Geometry check sheet. Reference: the model listing, model coordinates, mm. Coordinates: 2 decimals unless noted, no trailing zeros. Write each loop counter-clockwise with the first axis right and the second up, starting at its lowest first coordinate (ties: lowest second). Pieces come first, ordered by that corner, then holes. Notation, with made-up numbers: M 56,-0.5 L 77,-0.5 A18 ccw 77,18.5 Z; hole C -11,50 d8. An arc over 180 degrees is marked long. Put each result on its own line as item: value. Start each with the question number.
1) Scan lines: line 1 along Z through (x, y) = (10, -7.25); line 2 along Y through (x, z) = (6.25, 0); line 3 along Y through (x, z) = (7, 0). Record each from-to range of solid material in increasing order.
2) Cross-section at C-C on x = 2.5. Record the cut outline in (y, z), plus the area to 3 significant figures.
3) Gauge pin test, flat ends, axial feed: pin 1 (2 mm diameter, centred on x = 2.5, y = -6, fed in from -Z); pin 2 (3 mm diameter, centred on x = 7, y = -0.5, fed in from -Z); pin 3 (3 mm diameter, centred on x = 5.5, z = 8.5, fed in from -Y); pin 4 (6 mm diameter, centred on x = 7, y = -0.5, fed in from +Z). Record the tip position at first contact, or that the pin passes through.
4) Mould release check, pull along Z, two halves, no side actions. Record for faces 1 (the cylindrical face through (1.72, -2.656, 11.959)), 2 (the flat face through (0, -5, -8)), 3 (the cylindrical face through (6.076, 4.57, 7.167)): released by +Z, released by -Z, zero draft, split by the parting line, or undercut.
5) Cross-section at A-A on z = 0. Record the cut outline in (x, y).
Solid Edge part; units mm, degrees
sketch "Sketch1" plane through (0, 0, 0) normal (0, 0, 1) x (1, 0, 0)
  arc A0 (0, 9.1) -> (0.6, 8.5) centre (0.6, 9.1) ccw
  line L0 (0.6, 8.5) -> (11.4, 8.5)
  arc A1 (11.4, 8.5) -> (12, 9.1) centre (11.4, 9.1) ccw
  line L1 (12, 9.1) -> (12, 12.05)
  arc A2 (12, 12.05) -> (11.8, 12.25) centre (11.8, 12.05) ccw
  line L2 (11.8, 12.25) -> (8.7173, 12.25)
  arc A3 (8.7173, 12.25) -> (3.2827, 12.25) centre (6, 14.25) cw
  line L3 (3.2827, 12.25) -> (0.2, 12.25)
  arc A4 (0.2, 12.25) -> (0, 12.05) centre (0.2, 12.05) ccw
  line L4 (0, 12.05) -> (0, 9.1)
revolve "RevolvedProtrusion1" add sketch "Sketch1" angle 360 about axis through (11.4, 0, 0) along (-1, 0, 0)
Answer key:
1. line 1: z = -9.87 to -4.44, 4.44 to 9.87
1. line 2: y = -10.89 to -8.5, 8.5 to 10.89
1. line 3: y = -11.03 to -8.5, 8.5 to 11.03
2. outline: C 0,0 d24.5; hole C 0,0 d17
2. area: 244 mm²
3. pin 1: stops at z = -11.18
3. pin 2: stops at z = -11.97
3. pin 3: stops at y = -8.47
3. pin 4: stops at z = 12.25
4. face 1: split by the parting line
4. face 2: zero draft
4. face 3: undercut
5. outline: M 0,-12.05 A0.2 ccw 0.2,-12.25 L 3.28,-12.25 A3.37 cw 8.72,-12.25 L 11.8,-12.25 A0.2 ccw 12,-12.05 L 12,-9.1 A0.6 ccw 11.4,-8.5 L 0.6,-8.5 A0.6 ccw 0,-9.1 Z; M 0,9.1 A0.6 ccw 0.6,8.5 L 11.4,8.5 A0.6 ccw 12,9.1 L 12,12.05 A0.2 ccw 11.8,12.25 L 8.72,12.25 A3.37 cw 3.28,12.25 L 0.2,12.25 A0.2 ccw 0,12.05 Z
